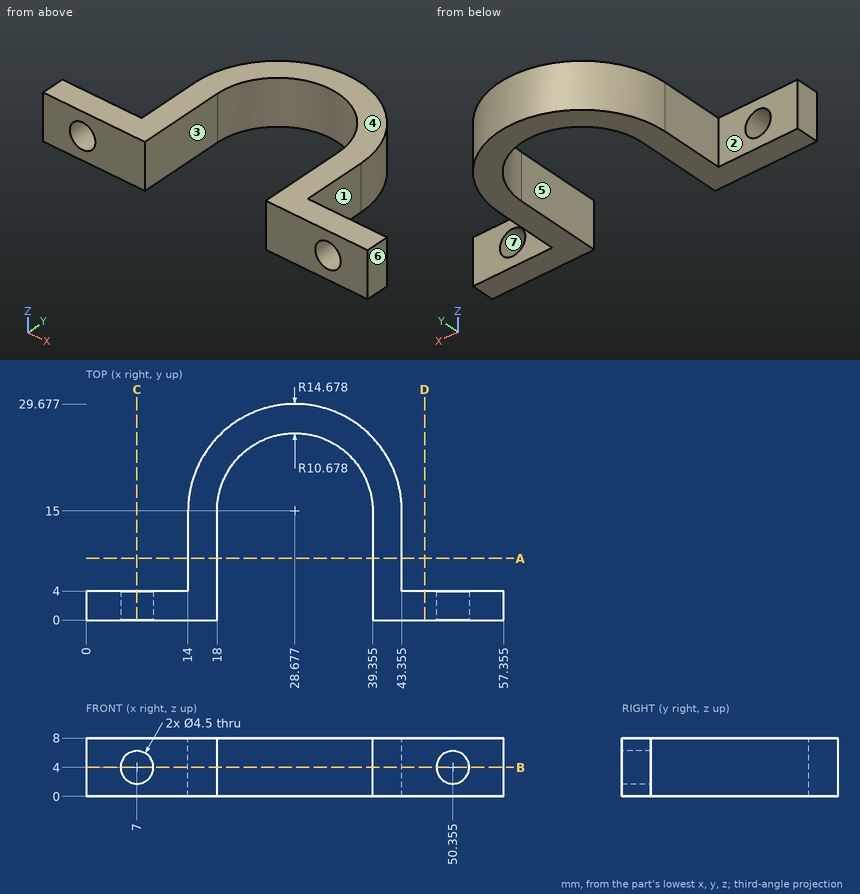
Here's the drawing with two shaded views (mm, measured from the low corner). I have some questions. A direction names the side the tool comes from. Give positions to 0.01 mm unless a question says otherwise; leave off trailing zeros. Loops run counter-clockwise (first coordinate to the right, second up) from the corner with the lowest first, then second, coordinate; pieces in that order, holes last. Notation, with made-up numbers: M 10.5,-26 L 57.5,-26 A10 ccw 57.5,-20 Z; hole C 43,11.5 d6. An arc over 180 degrees is marked long. One line per item, written item: value. Start each with the question number.
1) If we section it at B-B, the plane z = 4: Give the number of separate pieces and of enclosed holes in the cut face.
2) If we section it at A-A, the plane y = 8.5: Write out the boundary of the cut face in (x, z) (1 decimal), and give its area (3 significant figures).
3) I'm going to push flat-ended pins straight in: pin 1 (4 mm diameter, centred on x = 6.5, z = 4.5, fed in from +Y); pin 2 (2.5 mm diameter, centred on y = 6.5, z = 6, fed in from -X); pin 3 (4 mm diameter, centred on y = 24.5, z = 4.5, fed in from +X) (1 decimal). Where does each tip first touch, or does it pass through?
4) If I drill on line 1 (X direction, y = 4.25, z = 2.5) (1 decimal); line 2 (Y direction, x = 44, z = 1.75); line 3 (X direction, y = 3.5, z = 7) (1 decimal), over which ranges is the centre line in solid material (lowest first)? Write a range as [from, to].
5) Thinking about a two-plate mould opening in X: for the marked faces 4, 5, 6 and 7, which applies, +X half, -X half, draft (parallel to the pull), parting line (faces both ways), or undercut?
6) If we section it at D-D, the plane x = 46.5: Write out the boundary of the cut face in (y, z).
7) On a 3-axis mill with a long thin cutter (end or side, diameter ignored), from which of +Z, -Z, +X, -X, +Y, -Y can I reach the whole of each face in a straight line? I mean the marked faces 1, 2 and 3. Say none if no direction works.
8) If we section it at C-C, the plane x = 7: Write out the boundary of the cut face in (y, z).
Completed:
1. separate pieces: 3
1. enclosed holes: 0
2. outline: M 14,0 L 18,0 L 18,8 L 14,8 Z; M 39.4,0 L 43.4,0 L 43.4,8 L 39.4,8 Z
2. area: 64.0 mm^2
3. pin 1: stops at y = 4
3. pin 2: stops at x = 14
3. pin 3: stops at x = 41.3
4. line 1: x = [14, 18], [39.4, 43.4]
4. line 2: y = [0, 4]
4. line 3: x = [0, 18], [39.4, 57.4]
5. face 4: draft
5. face 5: undercut
5. face 6: +X half
5. face 7: undercut
6. outline: M 0,0 L 4,0 L 4,8 L 0,8 Z
7. face 1: +Z, -Z, +X, +Y
7. face 2: +Z, -Z, -X, +Y
7. face 3: +Z, -Z, -Y
8. outline: M 0,0 L 4,0 L 4,1.75 L 0,1.75 Z; M 0,6.25 L 4,6.25 L 4,8 L 0,8 Z
